Read the model definition and answer for the solid it produces. Units are mm, in the model's axes. A direction names the side the tool comes from. Round coordinates to 2 decimals unless told otherwise and drop trailing zeros. Write each loop counter-clockwise with the first axis right and the second up, starting at its lowest first coordinate (ties: lowest second). Pieces come first, ordered by that corner, then holes. Notation, with made-up numbers: (88.5, 8) - (92.5, 8) arc R20 ccw to (92.5, 43) - close; hole circle Ø1 at (19, 20.5). An arc over 180 degrees is marked (long way). One line per item, written item: value. Start each with the question number.
(1) A cutting plane is placed at D-D, the plane z = -1. Determine the outline of the cut face in (x, y) (3 decimals).
(2) A cutting plane is placed at A-A, the plane x = 0. Determine the outline of the cut face in (y, z) (1 decimal), plus the area to 3 significant figures.
(3) A cutting plane is placed at B-B, the plane z = -6.75. Determine the outline of the cut face in (x, y) (3 decimals).
(4) Flat-ended cylindrical pins translate along their axes: pin 1 Ø4 at (x, z) = (40.5, -1.5) entering from +Y; pin 2 Ø7.5 at (x, z) = (-40.5, -3.5) entering from -Y; pin 3 Ø5 at (x, z) = (52.5, 3) entering from -Y; pin 4 Ø1 at (y, z) = (-7.5, -6) entering from -X. Find the tip coordinate at first contact, or state that the pin passes through.
(5) Find the intervals of material crossed by L1, parallel to Y at x = 50.8, z = 2.85; L2, parallel to Z at x = 0, y = -18 (1 decimal); L3, parallel to X at y = -4, z = -5.25, in increasing order.
(6) The mould has two halves that part along X. Classify faces 1 (the face through (42, -1.905, -4)), 2 (the face through (57.15, -9, 2)), 3 (the face through (37.51, -9.63, -1.32)): +X half, -X half, draft (parallel to the pull), parting line (faces both ways), or undercut.
(7) For faces 4 (the face through (-10.883, -12.522, -1.432)), 5 (the face through (-44.45, -10, -5)), 6 (the face through (42, -17.145, -4)), 7 (the face through (-42, -17.145, -4)), determine the directions among +Z, -Z, +X, -X, +Y, -Y from which every point of the face is accessible in a straight line to the end or side of a thin tool.
(8) A cutting plane is placed at C-C, the plane x = -50.8. Determine the outline of the cut face in (y, z), plus the area to 3 significant figures.
from build123d import *

# Parameters (mm, degrees)
BOSS_EXTRUDE5_DEPTH         = 4.7625
F_11_0_191_DIAMETER_HOLE1_D = 4.8514
BOSS_EXTRUDE6_DEPTH         = 25.4
CUT_EXTRUDE1_DEPTH          = 65.15150159
CUT_EXTRUDE1_DEPTH_BACK     = 65.15150159
SKETCH7_R                   = 4.7625
FILLET2_R                   = 4.7625
BOSS_EXTRUDE7_DEPTH         = 7.62


with BuildPart() as part:
    # Sketch3 → Boss-Extrude5 (new body)
    with BuildSketch(Plane.XY):
        Polygon((-57.15, 0), (57.15, 0), (57.15, -19.05), (44.45, -19.05), (9.525, -25.4), (-9.525, -25.4), (-44.45, -19.05), (-57.15, -19.05), align=None)
    extrude(amount=BOSS_EXTRUDE5_DEPTH)

    # #11 (0.191) Diameter Hole1 (through all)
    with Locations(Plane(origin=(50.8, -9.525, 4.7625), x_dir=(1, 0, 0), z_dir=(0, 0, 1))):
        with Locations((0, 0), (-101.6, 0)):
            Hole(F_11_0_191_DIAMETER_HOLE1_D / 2)

    # Sketch6 → Boss-Extrude6 (add)
    with BuildSketch(Plane.XZ.offset(25.4)):
        with BuildLine():
            Line((9.525, 0), (9.525, -4.7625))
            ThreePointArc((9.525, -4.7625), (0, -14.2875), (-9.525, -4.7625))
            Line((-9.525, -4.7625), (-9.525, 0))
            Line((-9.525, 0), (9.525, 0))
        make_face()
    extrude(amount=-BOSS_EXTRUDE6_DEPTH)

    # Sketch7 → Cut-Extrude1 (cut, two sides: drawn at the far end of the back side and taken through both)
    with BuildSketch(Plane.XZ.offset(25.4).offset(-CUT_EXTRUDE1_DEPTH_BACK)):
        with Locations((0, -4.7625)):
            Circle(SKETCH7_R)
    extrude(amount=CUT_EXTRUDE1_DEPTH + CUT_EXTRUDE1_DEPTH_BACK, mode=Mode.SUBTRACT)

    # Fillet2
    fillet2_edges = [part.edges().sort_by_distance(p)[0] for p in [
        (-9.525, -12.7, 0),
        (9.525, -12.7, 0),
    ]]
    fillet(fillet2_edges, radius=FILLET2_R - 0.0001)  # a hair under: the kernel refuses the full size

    # Sketch8 → Boss-Extrude7 (add, symmetric)
    with BuildSketch(Plane(origin=(0, -9.525, 0), x_dir=(-1, 0, 0), z_dir=(0, -1, 0))):
        with BuildLine():
            Line((-44.45, 0), (-44.45, 9.525))
            Line((-44.45, 9.525), (-43.723723681, 9.525))
            ThreePointArc((-43.723723681, 9.525), (-40.249716578, 8.02021099), (-38.971047095, 4.45676888))
            ThreePointArc((-38.971047095, 4.45676888), (-37.476081499, 1.288492897), (-34.218370509, 0))
            Line((-34.218370509, 0), (-44.45, 0))
        make_face()
    boss_extrude7 = extrude(amount=BOSS_EXTRUDE7_DEPTH, both=True)

    # Mirror1: Boss-Extrude7 across plane
    add(boss_extrude7.mirror(Plane(origin=(0, 0, 0), x_dir=(0, 0, 1), z_dir=(1, 0, 0))))


solid = part.part
Here are the results:
1. outline: (-44.45, -17.145) - (-37.138, -17.145) - (-37.138, -1.905) - (-44.45, -1.905) - close; (-11.368, -25.065) - (-9.525, -25.4) - (-2.92, -25.4) - (-2.92, 0) - (-11.368, 0) - close; (2.92, -25.4) - (9.525, -25.4) - (11.368, -25.065) - (11.368, 0) - (2.92, 0) - close; (37.138, -17.145) - (44.45, -17.145) - (44.45, -1.905) - (37.138, -1.905) - close
2. outline: (-25.4, -14.3) - (0, -14.3) - (0, -9.5) - (-25.4, -9.5) - close; (-25.4, 0) - (0, 0) - (0, 4.8) - (-25.4, 4.8) - close
2. area: 242 mm²
3. outline: (-44.45, -17.145) - (-39.396, -17.145) - (-39.396, -1.905) - (-44.45, -1.905) - close; (-9.315, -25.4) - (-4.328, -25.4) - (-4.328, 0) - (-9.315, 0) - close; (4.328, -25.4) - (9.315, -25.4) - (9.315, 0) - (4.328, 0) - close; (39.396, -17.145) - (44.45, -17.145) - (44.45, -1.905) - (39.396, -1.905) - close
4. pin 1: y = 0
4. pin 2: y = -20.01
4. pin 3: y = -19.05
4. pin 4: x = -44.45
5. L1: -19.05 to -11.95, -7.1 to 0
5. L2: -14.3 to -9.5, 0 to 4.8
5. L3: -44.45 to -38.99, -9.51 to -4.74, 4.74 to 9.51, 38.99 to 44.45
6. face 1: draft
6. face 2: +X half
6. face 3: undercut
7. face 4: -Z, +Y, -Y
7. face 5: -Z, -X, +Y, -Y
7. face 6: -Z, +X, -Y
7. face 7: -Z, -X, -Y
8. outline: (-19.05, 0) - (-11.95, 0) - (-11.95, 4.76) - (-19.05, 4.76) - close; (-7.1, 0) - (0, 0) - (0, 4.76) - (-7.1, 4.76) - close
8. area: 67.6 mm²
